Part model, mm, in its own coordinate system. Give positions to 0.01 mm unless a question says otherwise; leave off trailing zeros. Order: outer loops, then holes, each group sorted by start corner. A loop starts at its lowest first (then second) coordinate and runs counter-clockwise, first axis right, second up.
1. Drop flat-ended pins along their axis: pin 1 Ø3 at (x, y) = (-50.5, -2.5) entering from +Z; pin 2 Ø1 at (y, z) = (7.5, -71.5) entering from -X; pin 3 Ø2 at (x, z) = (-31, -40) entering from -Y. Give the stop position or say it passes through.
2. Slice it at A-A on x = 27. List the corners of the cut face in (y, z), and give its area (3 significant figures).
3. Slice it at B-B on y = -14. List the corners of the cut face in (x, z), and give its area (3 significant figures).
4. Slice it at C-C on z = -12. List the corners of the cut face in (x, y), and give its area (3 significant figures).
5. Slice it at D-D on y = -41. List the corners of the cut face in (x, z).
6. Probe line 1 (Y direction, x = -31.5, z = -28); line 2 (Y direction, x = -33.5, z = -40); line 3 (X direction, y = 3, z = -8.5). List the from-to ranges inside material, lowest first.
from build123d import *

# Parameters (mm, degrees)
F3_SCALE = 2


with BuildPart() as f2:
    # F1 (on Front) → F2 (revolve)
    with BuildSketch(Plane.XZ):
        with BuildLine():
            Line((19.05, -41.2325449288), (25.4, -41.2325449288))
            ThreePointArc((25.4, -41.2325449288), (24.7856075246, -35.6797384638), (22.9721527844, -30.3955621177))
            ThreePointArc((22.9721527844, -30.3955621177), (34.1090092284, -16.9760269043), (38.1, 0))
            Line((38.1, 0), (31.75, 0))
            ThreePointArc((31.75, 0), (22.4506403027, -22.4506403027), (0, -31.75))
            Line((0, -31.75), (0, -38.1))
            ThreePointArc((0, -38.1), (9.0313967854, -37.0141036918), (17.5479819998, -33.8183134963))
            ThreePointArc((17.5479819998, -33.8183134963), (18.6707198187, -37.4501222327), (19.05, -41.2325449288))
        make_face()
    revolve(axis=Axis((0, 0, 1.3704523444), (0, 0, -1)))


with BuildPart() as f2_1:
    # F3: moved
    add(f2.part.scale(F3_SCALE))


solid = f2_1.part
Data:
1. pin 1: stops at z = -36.36
1. pin 2: stops at x = -49.16
1. pin 3: stops at y = -57.84
2. outline: (-71.26, 0) arc R71.26 ccw to (-37.17, -60.79) arc R43.03 ccw to (-43.03, -82.47) - (-26.88, -82.47) arc R26.88 cw to (-22.42, -67.64) arc R71.26 ccw to (22.42, -67.64) arc R26.88 cw to (26.88, -82.47) - (43.03, -82.47) arc R43.03 ccw to (37.17, -60.79) arc R71.26 ccw to (71.26, 0) - (57.47, 0) arc R57.47 cw to (-57.47, 0) - close
2. area: 3,400 mm2
3. outline: (-74.9, 0) arc R74.9 ccw to (-43.76, -60.79) arc R48.83 ccw to (-48.83, -82.47) - (-35.43, -82.47) arc R35.43 cw to (-32.18, -67.64) arc R74.9 ccw to (32.18, -67.64) arc R35.43 cw to (35.43, -82.47) - (48.83, -82.47) arc R48.83 ccw to (43.76, -60.79) arc R74.9 ccw to (74.9, 0) - (61.94, 0) arc R61.94 cw to (-61.94, 0) - close
3. area: 3,290 mm2
4. outline: circle Ø150.5 at (0, 0); hole circle Ø124.71 at (0, 0)
4. area: 5,570 mm2
5. outline: (-64.23, 0) arc R64.23 ccw to (-20.73, -60.79) arc R29.99 ccw to (-29.99, -82.47) - (29.99, -82.47) arc R29.99 ccw to (20.73, -60.79) arc R64.23 ccw to (64.23, 0) - (48.49, 0) arc R48.49 cw to (-48.49, 0) - close
6. line 1: y = -63.48 to -47.5, 47.5 to 63.48
6. line 2: y = -55.54 to -36.19, 36.19 to 55.54
6. line 3: x = -75.66 to -62.86, 62.86 to 75.66
